Could you check a few things on this model? Use its own coordinates, in mm. Face numbers are marked on the shaded views. A direction names the side the tool comes from. Coordinates: 2 decimals unless noted, no trailing zeros. Write each loop counter-clockwise with the first axis right and the second up, starting at its lowest first coordinate (ties: lowest second). Pieces come first, ordered by that corner, then holes.
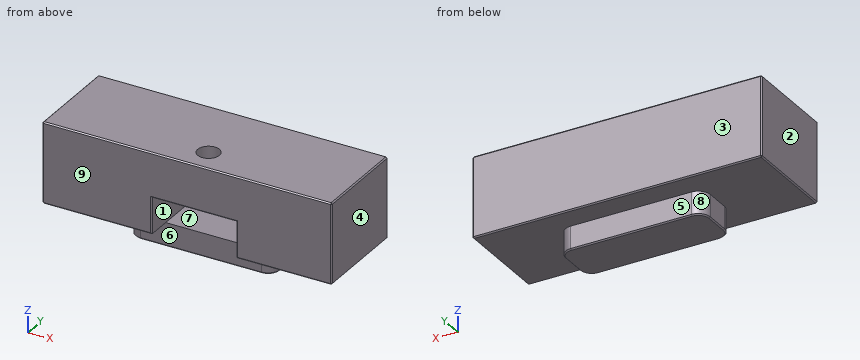
```python
from build123d import *

# Parameters (mm, degrees)
F0_W     = 120
F0_H     = 33.5
F1_DEPTH = 40
F4_DEPTH = 9.7
F5_R     = 4.5
F6_DEPTH = 33.5
F7_W     = 35
F7_H     = 15
F8_DEPTH = 29
F9_SIZE  = 0.5
F10_SIZE = 0.5


with BuildPart() as f1:
    # F0 (on Front) → F1 (new body)
    with BuildSketch(Plane.XZ):
        with Locations((-2.857143, 0)):
            Rectangle(F0_W, F0_H)
    extrude(amount=-F1_DEPTH)

    # F3 (on face) → F4 (join)
    with BuildSketch(Plane(origin=(0, 0, -16.75), x_dir=(1, 0, 0), z_dir=(0, 0, -1))):
        with BuildLine():
            ThreePointArc((27.142857, -15), (25.678391, -11.464466), (22.142857, -10))
            Line((22.142857, -10), (-27.857143, -10))
            ThreePointArc((-27.857143, -10), (-31.392677, -11.464466), (-32.857143, -15))
            Line((-32.857143, -15), (-32.857143, -25))
            ThreePointArc((-32.857143, -25), (-31.392677, -28.535534), (-27.857143, -30))
            Line((-27.857143, -30), (22.142857, -30))
            ThreePointArc((22.142857, -30), (25.678391, -28.535534), (27.142857, -25))
            Line((27.142857, -25), (27.142857, -15))
        make_face()
    extrude(amount=F4_DEPTH)

    # F5 (on face) → F6 (cut)
    with BuildSketch(Plane.XY.offset(16.75)):
        with Locations((0, 10.5)):
            Circle(F5_R)
    extrude(amount=-F6_DEPTH, mode=Mode.SUBTRACT)

    # F7 (on face) → F8 (cut)
    with BuildSketch(Plane.XZ):
        with Locations((0, -9.25)):
            Rectangle(F7_W, F7_H)
    extrude(amount=-F8_DEPTH, mode=Mode.SUBTRACT)

    # F9
    f9_edges = [f1.edges().sort_by_distance(p)[0] for p in [
        (-2.857143, 0, 16.75),
        (57.142857, 20, 16.75),
        (-2.857143, 40, 16.75),
        (-62.857143, 20, 16.75),
        (-62.857143, 0, 0),
        (57.142857, 0, 0),
        (57.142857, 40, 0),
        (-62.857143, 40, 0),
        (-62.857143, 20, -16.75),
        (-40.178572, 0, -16.75),
        (37.321428, 0, -16.75),
        (-17.5, 0, -9.25),
        (0, 0, -1.75),
        (17.5, 0, -9.25),
        (57.142857, 20, -16.75),
        (-2.857143, 40, -16.75),
    ]]
    chamfer(f9_edges, length=F9_SIZE)

    # F10
    f10_edges = [f1.edges().sort_by_distance(p)[0] for p in [
        (-2.857143, 10, -26.45),
    ]]
    chamfer(f10_edges, length=F10_SIZE)


solid = f1.part
```
1. Please list where these lines run through material, in increasing order: line 1 along X through (y, z) = (13.5, -15.5); line 2 along Z through (x, y) = (-9, 18); line 3 along Y through (x, z) = (0, 11).
Verdict:
line 1: x = -62.86 to -17.5, 17.5 to 57.14
line 2: z = -26.45 to -16.75, -1.75 to 16.75
line 3: y = 0 to 6, 15 to 40
2. I want a section at A-A on x = 0. Please give me the cut outline in (y, z).
Verdict:
outline: (0, -1.25) - (0.5, -1.75) - (6, -1.75) - (6, 16.75) - (0.5, 16.75) - (0, 16.25) - close; (10, -25.95) - (10.5, -26.45) - (29.5, -26.45) - (30, -25.95) - (30, -16.75) - (39.5, -16.75) - (40, -16.25) - (40, 16.25) - (39.5, 16.75) - (15, 16.75) - (15, -1.75) - (29, -1.75) - (29, -16.75) - (10, -16.75) - close
3. I want a section at C-C on z = -19. Please give me the cut outline in (x, y), plus the area to 3 significant figures.
Verdict:
outline: (-32.86, 15) arc R5 ccw to (-27.86, 10) - (22.14, 10) arc R5 ccw to (27.14, 15) - (27.14, 25) arc R5 ccw to (22.14, 30) - (-27.86, 30) arc R5 ccw to (-32.86, 25) - close
area: 1,180 mm2
4. I want a section at B-B on y = 37. Please give me the cut outline in (x, z), plus the area to 3 significant figures.
Verdict:
outline: (-62.86, -16.25) - (-62.36, -16.75) - (56.64, -16.75) - (57.14, -16.25) - (57.14, 16.25) - (56.64, 16.75) - (-62.36, 16.75) - (-62.86, 16.25) - close
area: 4,020 mm2
5. If we mould it in two halves opening along X, with no side actions, what happens to the marked faces 1, 2, 3 and 4? For each: pulls with the +X half, pulls with the -X half, needs draft (parallel to the pull), parting line crosses it, or undercut.
Verdict:
face 1: undercut
face 2: pulls with the -X half
face 3: needs draft
face 4: pulls with the +X half
6. For pin 1 (5 mm diameter, centred on x = -30, z = -18.5, fed in from -Y); pin 2 (7.5 mm diameter, centred on x = 6.5, z = -20.5, fed in from -Y); pin 3 (7.5 mm diameter, centred on x = 2.5, z = -12.5, fed in from -Y); pin 4 (7.5 mm diameter, centred on y = 20, z = -22, fed in from +X), each with a flat end and sliding along its axis, tell me the tip position at first contact or that it passes through.
Verdict:
pin 1: stops at y = 0
pin 2: stops at y = 10
pin 3: stops at y = 29
pin 4: stops at x = 27.14
7. On a 3-axis mill with a long thin cutter (end or side, diameter ignored), from which of +Z, -Z, +X, -X, +Y, -Y can I reach the whole of each face in a straight line? I mean the marked faces 5, 6, 7, 8 and 9. Say none if no direction works.
Verdict:
face 5: -Z, +X, -X, +Y
face 6: -Z, +X, -X, -Y
face 7: -Y
face 8: -Z, -X, +Y
face 9: +Z, -Z, +X, -X, -Y
